The figure shows three views and two pictorial views of one solid part (mm, origin at its lowest corner). Answer the questions. A direction names the side the tool comes from. Coordinates: 2 decimals unless noted, no trailing zeros. Order: outer loops, then holes, each group sorted by start corner. A loop starts at its lowest first (then second) coordinate and runs counter-clockwise, first axis right, second up. Notation, with made-up numbers: (29, -34) -> (72, -34) arc R22 ccw to (72, -13) -> close; hole circle Ø6 at (27.5, 4.25). An arc over 180 degrees is marked (long way). Use one line per item in the form item = value.
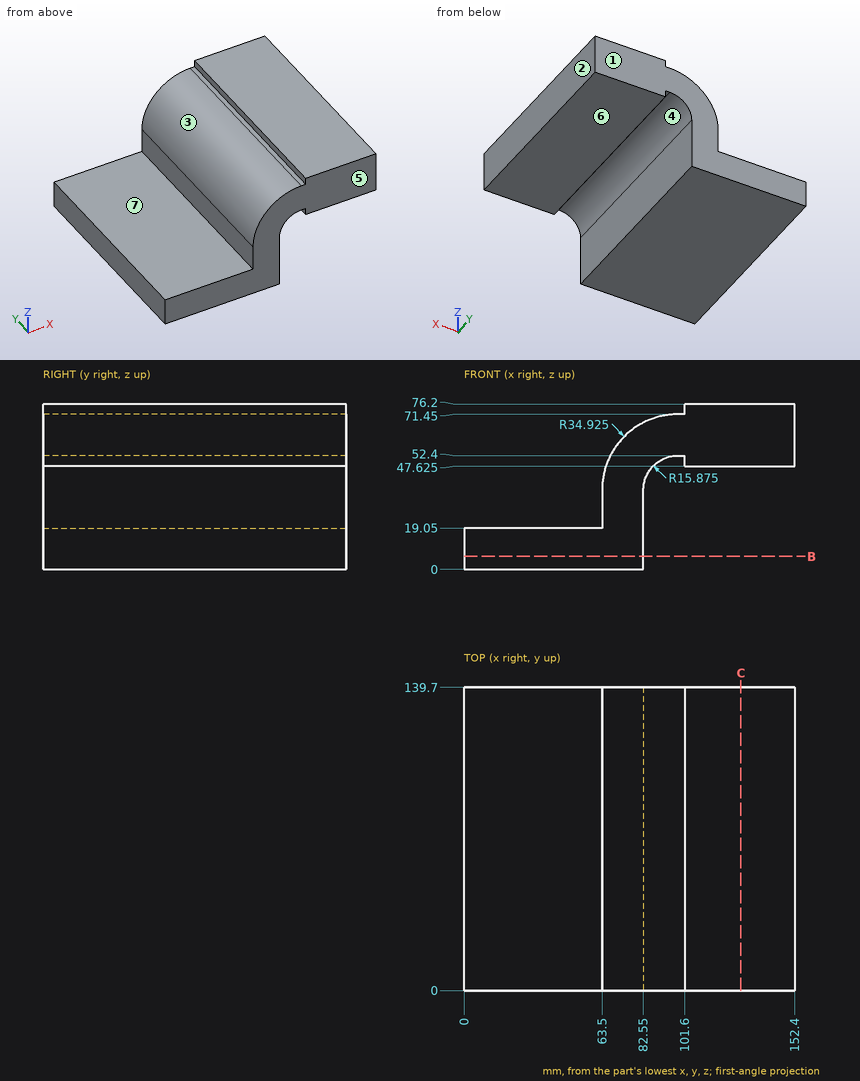
(1) Straight lines are drawn through the part: line 1 along X through (y, z) = (39.5, 31); line 2 along Z through (x, y) = (32, 39.5); line 3 along Z through (x, y) = (115.5, 55.5) (3 decimals). For each, find the intervals that lie inside material, in ascending order.
Data:
line_1 = 63.5 to 82.55
line_2 = 0 to 19.05
line_3 = 47.625 to 76.2
(2) Which of the six approach directions +Z, -Z, +X, -X, +Y, -Y give full straight-line access (tool end or side, diameter ignored) to the marked faces 5, 6 and 7?
Data:
face_5 = +Z, -Z, +X, -X, -Y
face_6 = -Z, +X, +Y, -Y
face_7 = +Z, -X, +Y, -Y
(3) Section C-C on x = 127.5 is taken. Write down the section's boundary in (y, z) (3 decimals).
Data:
outline = (0, 47.625) -> (139.7, 47.625) -> (139.7, 76.2) -> (0, 76.2) -> close
(4) Each of these flat-tipped pins is pushed along its axis until it touches: P1, Ø1.4, axis at y = 55.5, z = 73, coming from the -X side; P2, Ø2.5, axis at x = 100.5, y = 93.5, coming from the -Z side (3 decimals); P3, Ø1, axis at y = 80.5, z = 25.5, coming from the -X side. Where does it stop, or does it pass through?
Data:
P1 = 101.6
P2 = 47.625
P3 = 63.5
(5) Section B-B on z = 6 is taken. Write down the section's boundary in (x, y).
Data:
outline = (0, 0) -> (82.55, 0) -> (82.55, 139.7) -> (0, 139.7) -> close
(6) The mould has two halves that part along X. Classify the marked faces 1, 2, 3 and 4: released by +X, released by -X, zero draft, split by the parting line, or undercut.
Data:
face_1 = zero draft
face_2 = released by +X
face_3 = released by -X
face_4 = undercut
